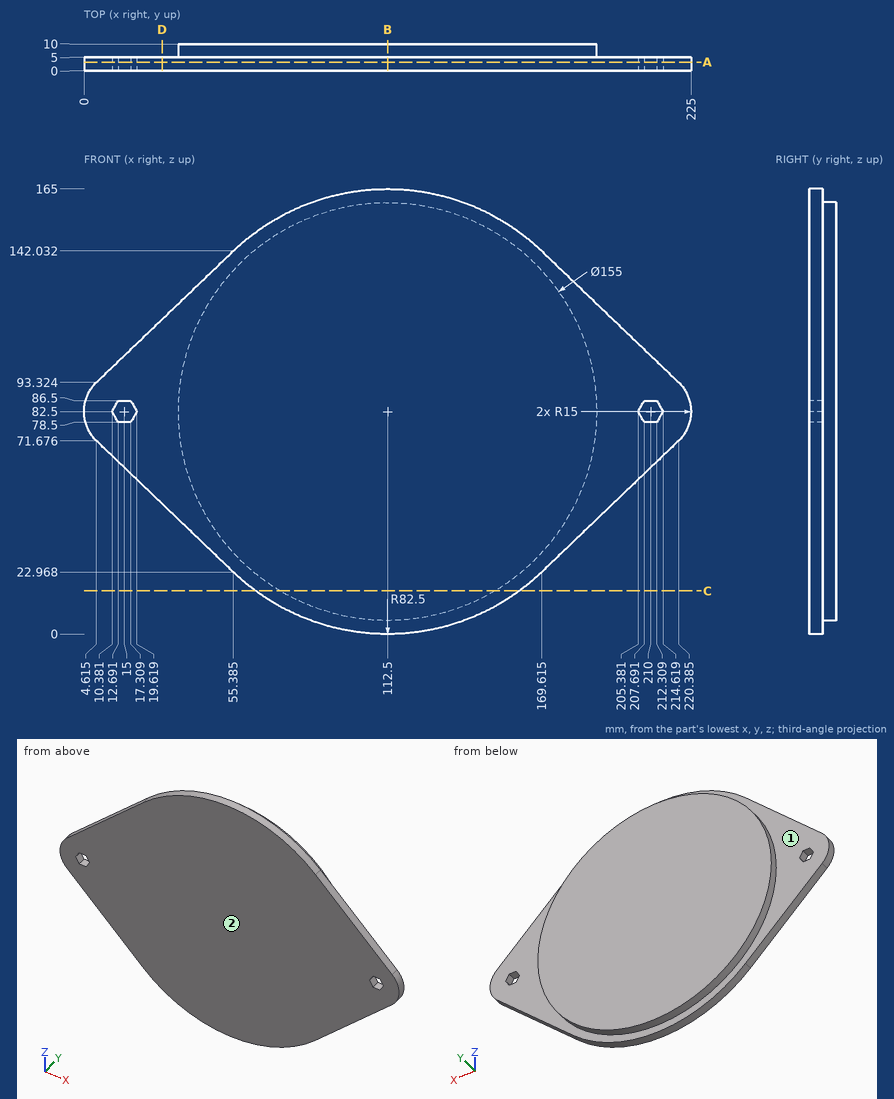
Design review of the part shown in the three views and the two pictorial views. Dimensions are in mm from the part's minimum x, y and z. A direction names the side the tool comes from. Coordinates: 2 decimals unless noted, no trailing zeros. Order: outer loops, then holes, each group sorted by start corner. A loop starts at its lowest first (then second) coordinate and runs counter-clockwise, first axis right, second up.
1) Clearance check with flat-ended pins moving along their axes: pin 1 (2.5 mm diameter, centred on x = 211, y = 3.5, fed in from -Z); pin 2 (4 mm diameter, centred on x = 182, y = 3.5, fed in from +Z); pin 3 (2.5 mm diameter, centred on x = 210, y = 3.5, fed in from +Z) (1 decimal). State where each tip first meets the part, or that it passes through.
2) Take a section at B-B, the plane x = 112.5. Give the boundary of the cut face in (y, z).
3) Take a section at C-C, the plane z = 16. Give the boundary of the cut face in (x, y).
4) Wall thickness on line 1 along Y through (x, z) = (79, 155); line 2 along X through (y, z) = (1, 153.5) (1 decimal); line 3 along Z through (x, y) = (204, 2.5) (1 decimal): over which ranges is each line inside the solid? List them lowest first.
5) Take a section at A-A, the plane y = 3.25. Give the boundary of the cut face in (x, z) (1 decimal).
6) Take a section at D-D, the plane x = 29. Give the boundary of the cut face in (y, z), and give its area (3 significant figures).
7) For the marked faces 1 and 2, list the 3-axis set-ups (+Z, -Z, +X, -X, +Y, -Y) from which the entire face can be reached by the end or side of a thin tool; tool diameter is ignored.
Returned:
1. pin 1: stops at z = 61.47
1. pin 2: stops at z = 132.07
1. pin 3: stops at z = 104.5
2. outline: (0, 0) - (5, 0) - (5, 5) - (10, 5) - (10, 160) - (5, 160) - (5, 165) - (0, 165) - close
3. outline: (63.67, 0) - (161.33, 0) - (161.33, 5) - (152.3, 5) - (152.3, 10) - (72.7, 10) - (72.7, 5) - (63.67, 5) - close
4. line 1: y = 0 to 5
4. line 2: x = 70.5 to 154.5
4. line 3: z = 56 to 109
5. outline: (4.6, 71.7) - (55.4, 23) arc R82.5 ccw to (169.6, 23) - (220.4, 71.7) arc R15 ccw to (220.4, 93.3) - (169.6, 142) arc R82.5 ccw to (55.4, 142) - (4.6, 93.3) arc R15 ccw to start; hole (10.4, 82.5) - (12.7, 78.5) - (17.3, 78.5) - (19.6, 82.5) - (17.3, 86.5) - (12.7, 86.5) - close; hole (205.4, 82.5) - (207.7, 78.5) - (212.3, 78.5) - (214.6, 82.5) - (212.3, 86.5) - (207.7, 86.5) - close
6. outline: (0, 48.28) - (5, 48.28) - (5, 116.72) - (0, 116.72) - close
6. area: 342 mm2
7. face 1: +Y
7. face 2: +Z, -Z, +X, -X, -Y
